Verification items for this drawing (mm, ordinates from the low corner). A direction names the side the tool comes from. Round coordinates to 2 decimals unless told otherwise and drop trailing zeros. Loops run counter-clockwise (first coordinate to the right, second up) from the corner with the lowest first, then second, coordinate; pieces in that order, holes last. Notation, with made-up numbers: M 32,-11 L 38,-11 A13 ccw 38,-4 Z; hole C 17,3 d10. An arc over 180 degrees is marked long. Use one line per item in the form item = value. Start each with the question number.
1. Draft check along X on the marked faces 1, 2 and 3. Enter one of: pulls with the +X half, pulls with the -X half, needs draft (parallel to the pull), parting line crosses it, or undercut.
2. Set-up check for the marked faces 4 and 5: record each of +Z, -Z, +X, -X, +Y, -Y from which the full face is reachable in a straight line by a thin tool's end or side.
3. Cross-section at C-C (y = 9.25). Record the boundary of the cut face in (x, z).
4. Cross-section at B-B (z = 5). Record the boundary of the cut face in (x, y).
5. Material ranges on line 1 (Y direction, x = 4.5, z = 5.5); line 2 (Y direction, x = 7.75, z = 6.5); line 3 (X direction, y = 1.75, z = 9), recorded low to high.
6. Go/stop test with flat-tipped pins: pin 1 (2.5 mm diameter, centred on x = 4, z = 4.5, fed in from -Y); pin 2 (1 mm diameter, centred on y = 7, z = 3.5, fed in from +X); pin 3 (1.5 mm diameter, centred on y = 3, z = 6, fed in from +X). Record where each tip stops, or that it passes through.
7. Cross-section at A-A (y = 3). Record the boundary of the cut face in (x, z), then the cut area to 3 significant figures.
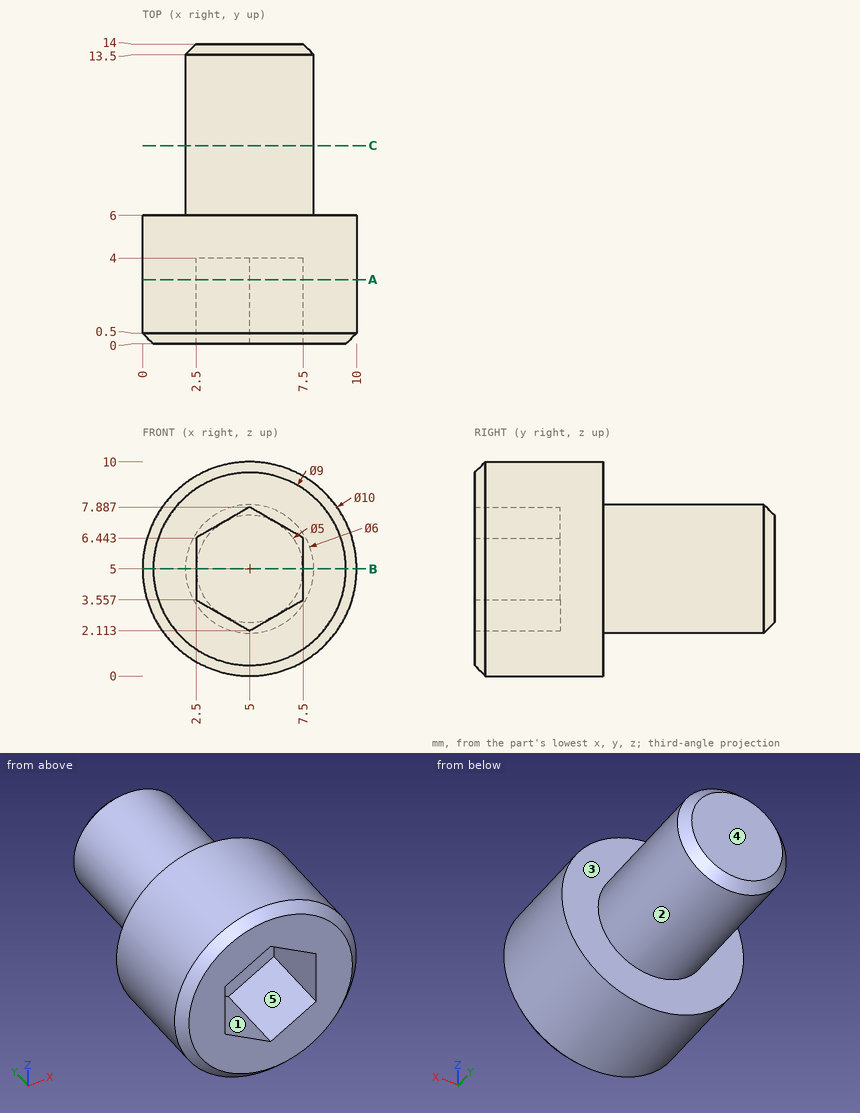
Reported:
q1.face_1 = undercut
q1.face_2 = parting line crosses it
q1.face_3 = needs draft
q2.face_4 = +Z, -Z, +X, -X, +Y
q2.face_5 = -Y
q3.outline = C 5,5 d6
q4.outline = M 0,0.5 L 0.5,0 L 2.5,0 L 2.5,4 L 7.5,4 L 7.5,0 L 9.5,0 L 10,0.5 L 10,6 L 8,6 L 8,13.5 L 7.5,14 L 2.5,14 L 2,13.5 L 2,6 L 0,6 Z
q5.line_1 = 4 to 14
q5.line_2 = 0 to 6
q5.line_3 = 2 to 8
q6.pin_1 = 4
q6.pin_2 = 7.83
q6.pin_3 = 9.99
q7.outline = C 5,5 d10; hole M 2.5,3.56 L 5,2.11 L 7.5,3.56 L 7.5,6.44 L 5,7.89 L 2.5,6.44 Z
q7.area = 56.9 mm²
